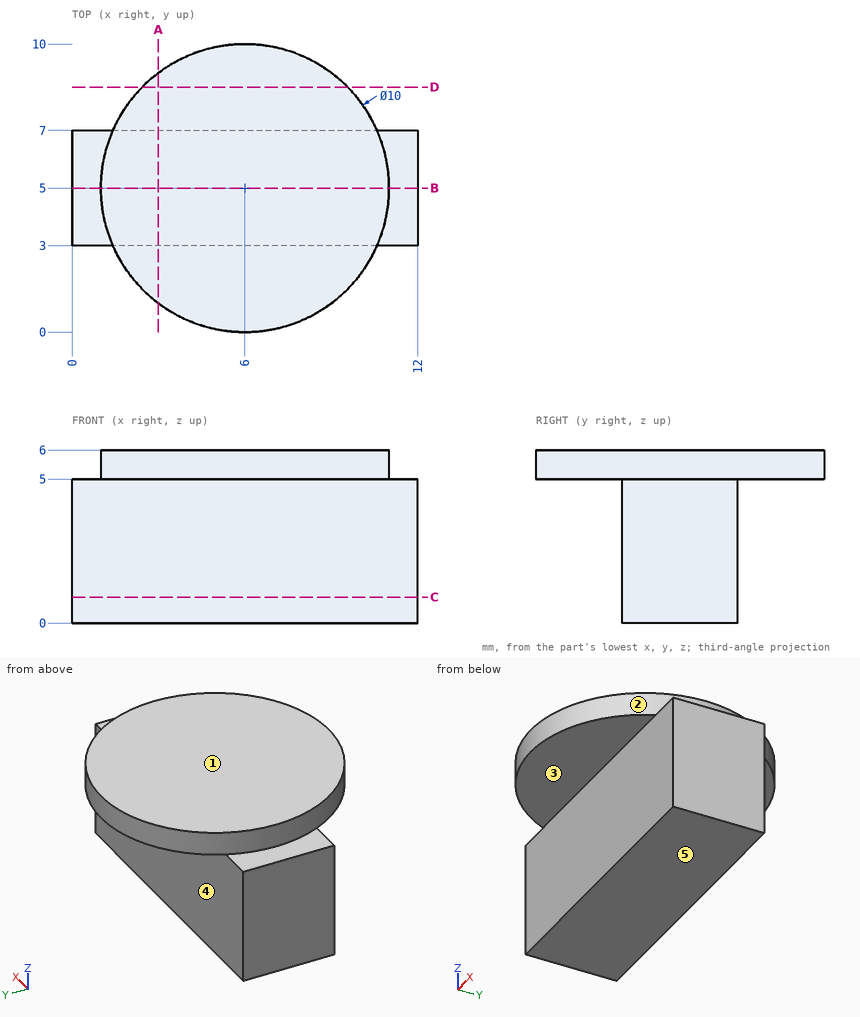
Here's the drawing with two shaded views (mm, measured from the low corner). I have some questions. A direction names the side the tool comes from. Coordinates: 2 decimals unless noted, no trailing zeros. Order: outer loops, then holes, each group sorted by start corner. A loop starts at its lowest first (then second) coordinate and runs counter-clockwise, first axis right, second up.
Item 1: I need wall thicknesses on line 1 (Y direction, x = 6.25, z = 4.45); line 2 (Z direction, x = 5.75, y = 1.5); line 3 (Z direction, x = 0.5, y = 3.25). Which ranges of each line are inside material? Lowest first, please.
Result sheet:
line 1: y = 3 to 7
line 2: z = 5 to 6
line 3: z = 0 to 5
Item 2: If we section it at C-C on z = 0.9: List the corners of the cut face in (x, y) for me.
Result sheet:
outline: (0, 3) - (12, 3) - (12, 7) - (0, 7) - close
Item 3: For P1, Ø2, axis at x = 4.5, z = 3.5, coming from the -Y side; P2, Ø1.5, axis at x = 3.5, y = 9, coming from the -Z side; P3, Ø0.7, axis at x = 0.5, y = 5, coming from the +Z side, each with a flat end and sliding along its axis, tell me the tip position at first contact or that it passes through.
Result sheet:
P1: stops at y = 3
P2: stops at z = 5
P3: stops at z = 5
Item 4: If we section it at A-A on x = 3: List the corners of the cut face in (y, z) for me.
Result sheet:
outline: (1, 5) - (3, 5) - (3, 0) - (7, 0) - (7, 5) - (9, 5) - (9, 6) - (1, 6) - close
Item 5: If we section it at B-B on y = 5: List the corners of the cut face in (x, z) for me.
Result sheet:
outline: (0, 0) - (12, 0) - (12, 5) - (11, 5) - (11, 6) - (1, 6) - (1, 5) - (0, 5) - close
Item 6: For the marked faces 1, 2, 3, 4 and 5, which set-ups out of +Z, -Z, +X, -X, +Y, -Y let a thin tool reach every point of the face, with its end or its side?
Result sheet:
face 1: +Z, +X, -X, +Y, -Y
face 2: +Z
face 3: -Z, +X, -X, -Y
face 4: -Z, +X, -X, +Y
face 5: -Z, +X, -X, +Y, -Y
Item 7: If we section it at D-D on y = 8.5: List the corners of the cut face in (x, z) for me, plus the area to 3 significant figures.
Result sheet:
outline: (2.43, 5) - (9.57, 5) - (9.57, 6) - (2.43, 6) - close
area: 7.14 mm2
